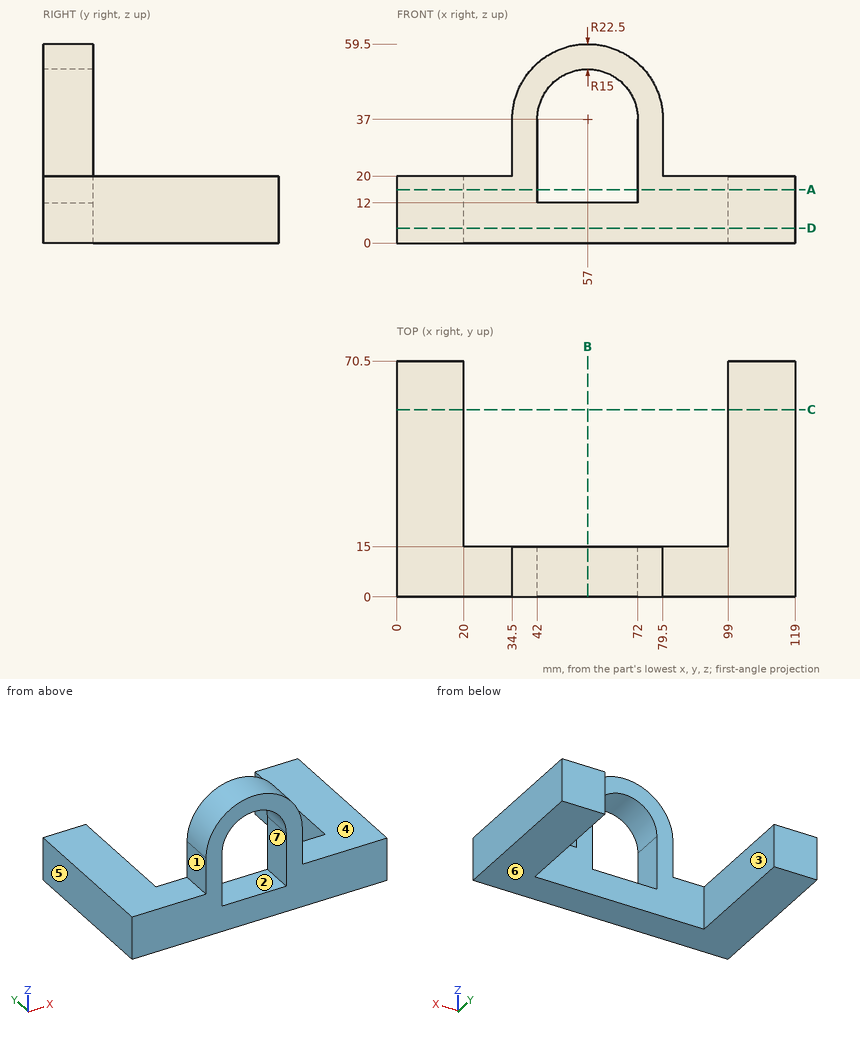
Input: dimensioned drawing with shaded views. Units: mm. Origin: part minimum x, y, z. A direction names the side the tool comes from. Give positions to 0.01 mm unless a question says otherwise; leave off trailing zeros. Loops run counter-clockwise (first coordinate to the right, second up) from the corner with the lowest first, then second, coordinate; pieces in that order, holes last. Notation, with made-up numbers: (54, 7.25) -> (60, 7.25) arc R17 cw to (60, 19.25) -> close; hole circle Ø9 at (70.5, 71.25). An arc over 180 degrees is marked (long way). Use a Markdown table: item, result. Add a question column.
1) Pull-direction query (X, two-part tool) for the marked faces 5, 6 and 7; classes: +X half, -X half, draft (parallel to the pull), parting line (faces both ways), or undercut.
2) Section query D-D, the plane z = 4.5. Return the cut outline in (x, y).
3) First-contact query: pin 1 (7.5 mm diameter, centred on x = 51.5, y = 6.5, fed in from +Z); pin 2 (16.5 mm diameter, centred on y = 9.5, z = 32.5, fed in from -X); pin 3 (12 mm diameter, centred on y = 8.5, z = 27.5, fed in from +X). Flat tips, straight axial feed; report the tip coordinate or a pass-through.
4) Section query B-B, the plane x = 57. Return the cut outline in (y, z), then the cut area to 4 significant figures.
5) Section query C-C, the plane y = 56. Return the cut outline in (x, z).
6) Line query: line 1 along X through (y, z) = (35, 17); line 2 along X through (y, z) = (10.5, 16); line 3 along Y through (x, z) = (48, 50). Output: solid intervals per line, ascending. Write a range as [from, to].
7) Reachability of the marked faces 1, 2, 3 and 4 from +Z, -Z, +X, -X, +Y, -Y: full face, straight path, thin tool, end or side. Return the list, or none.
8) Section query A-A, the plane z = 16. Return the cut outline in (x, y).
Numbers:
| question | item | result |
|---|---|---|
| 1 | face 5 | -X half |
| 1 | face 6 | draft |
| 1 | face 7 | undercut |
| 2 | outline | (0, 0) -> (119, 0) -> (119, 70.5) -> (99, 70.5) -> (99, 15) -> (20, 15) -> (20, 70.5) -> (0, 70.5) -> close |
| 3 | pin 1 | stops at z = 59.43 |
| 3 | pin 2 | stops at x = 34.5 |
| 3 | pin 3 | stops at x = 79.5 |
| 4 | outline | (0, 0) -> (15, 0) -> (15, 12) -> (0, 12) -> close; (0, 52) -> (15, 52) -> (15, 59.5) -> (0, 59.5) -> close |
| 4 | area | 292.5 mm2 |
| 5 | outline | (0, 0) -> (20, 0) -> (20, 20) -> (0, 20) -> close; (99, 0) -> (119, 0) -> (119, 20) -> (99, 20) -> close |
| 6 | line 1 | x = [0, 20], [99, 119] |
| 6 | line 2 | x = [0, 42], [72, 119] |
| 6 | line 3 | y = [0, 15] |
| 7 | face 1 | +Z, -X, +Y, -Y |
| 7 | face 2 | +Y, -Y |
| 7 | face 3 | +Z, -Z, +Y |
| 7 | face 4 | +Z, +X, +Y, -Y |
| 8 | outline | (0, 0) -> (42, 0) -> (42, 15) -> (20, 15) -> (20, 70.5) -> (0, 70.5) -> close; (72, 0) -> (119, 0) -> (119, 70.5) -> (99, 70.5) -> (99, 15) -> (72, 15) -> close |
